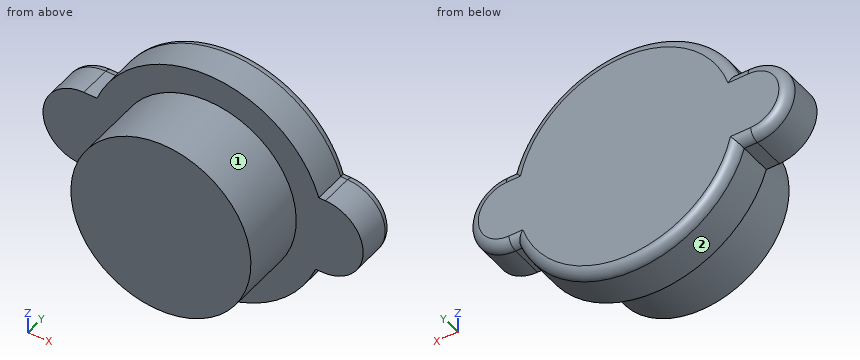
from build123d import *

# Parameters (mm, degrees)
SKETCH11_R = 18.415
NECK_DEPTH = 14.224
SKETCH12_R = 24.098503073
LID_DEPTH  = 8.89
FILLET3_R  = 2


with BuildPart() as part:
    # Sketch11 → neck (new body)
    with BuildSketch(Plane(origin=(0, 0, 0), x_dir=(1, 0, 0), z_dir=(0, 1, 0))):
        with Locations(Location((0, 0, 0), (0, 0, 270))):
            Circle(SKETCH11_R)
    extrude(amount=NECK_DEPTH)

    # Sketch12 → lid (add)
    with BuildSketch(Plane(origin=(0, 14.224, 0), x_dir=(1, 0, 0), z_dir=(0, 1, 0))):
        Circle(SKETCH12_R)
        with BuildLine():
            Line((-25.707660556, 6.978419473), (23.749239481, 9.0074205))
            ThreePointArc((23.749239481, 9.0074205), (32.097843424, 1.316834602), (24.407257526, -7.031769341))
            Line((24.407257526, -7.031769341), (-25.049642512, -9.060770368))
            ThreePointArc((-25.049642512, -9.060770368), (-33.398246454, -1.37018447), (-25.707660556, 6.978419473))
        make_face()
    extrude(amount=LID_DEPTH)

    # Fillet3
    fillet3_edges = [part.edges().sort_by_distance(p)[0] for p in [
        (-24.370076377, 23.114, -7.033294721),
        (23.061856817, 23.114, -8.979220186),
        (-0.98782558, 23.114, -24.078248504),
        (-33.398246454, 23.114, 1.37018447),
        (-23.712058333, 23.114, 9.00589512),
        (0.98782558, 23.114, 24.078248504),
        (23.719874862, 23.114, 7.059969655),
        (32.097843424, 23.114, -1.316834602),
    ]]
    fillet(fillet3_edges, radius=FILLET3_R)


solid = part.part
Build history of the part. All positions in model axes, mm. Face numbers are marked on the shaded views. A direction names the side the tool comes from. Coordinates: 2 decimals unless noted, no trailing zeros. Order: outer loops, then holes, each group sorted by start corner. A loop starts at its lowest first (then second) coordinate and runs counter-clockwise, first axis right, second up. Notation, with made-up numbers: (5, -30) - (63, -30) arc R9 cw to (63, -14) - close; hole circle Ø5 at (-13, 80). An arc over 180 degrees is marked (long way). Write item = value, one per line. Start each with the question number.
1) 3-axis set-ups, long thin cutter, end or side, ignore diameter. For the marked faces 1 and 2: which of +Z, -Z, +X, -X, +Y, -Y reach the whole face in a straight line?
2) Saw through at C-C on y = 6.5. Write the cut outline in (x, z) (3 decimals), then the cut area to 3 significant figures.
3) Wall check: line 1 along Y through (x, z) = (21.5, 4.5); line 2 along X through (y, z) = (6.25, 0) (3 decimals); line 3 along Z through (x, y) = (3, 5). Give the ranges that are in metal, low to high. Write a range as from..to.
4) Saw through at B-B on y = 16.25. Write the cut outline in (x, z), then the cut area to 3 significant figures.
5) Flat gauge pins, fed straight in: pin 1 Ø2 at (y, z) = (5.5, 5) entering from -X; pin 2 Ø3 at (x, z) = (18, 11.5) entering from -Y; pin 3 Ø8 at (x, z) = (5, 4) entering from -Y; pin 4 Ø10 at (x, y) = (-23.5, 13) entering from +Z. Where does each tip first touch, or does it go through?
6) Saw through at A-A on x = 0. Write the cut outline in (y, z) (1 decimal), then the cut area to 3 significant figures.
From the geometry:
q1.face_1 = -Y
q1.face_2 = -Z, +Y, -Y
q2.outline = circle Ø36.83 at (0, 0)
q2.area = 1,070 mm^2
q3.line_1 = 14.22..23.11
q3.line_2 = -18.415..18.415
q3.line_3 = -18.17..18.17
q4.outline = (-25.71, -6.98) - (-23.03, -7.09) arc R24.1 ccw to (22.37, -8.95) - (23.75, -9.01) arc R8.03 ccw to (24.41, 7.03) - (23.03, 7.09) arc R24.1 ccw to (-22.37, 8.95) - (-25.05, 9.06) arc R8.03 ccw to start
q4.area = 2,060 mm^2
q5.pin_1 = -17.98
q5.pin_2 = 14.22
q5.pin_3 = 0
q5.pin_4 = 15.26
q6.outline = (0, -18.4) - (14.2, -18.4) - (14.2, -24.1) - (21.1, -24.1) arc R2 ccw to (23.1, -22.1) - (23.1, 22.1) arc R2 ccw to (21.1, 24.1) - (14.2, 24.1) - (14.2, 18.4) - (0, 18.4) - close
q6.area = 951 mm^2
